```python
from build123d import *

# Parameters (mm, degrees)
F0_W      = 42
F0_H      = 31
F0_R      = 2.25
F0_W_2    = 32
F0_H_2    = 15
F1_DEPTH  = 7
F0_H_3    = 21
F2_DEPTH  = 3
F0_H_4    = 19
F3_DEPTH  = 17
F4_R      = 5
F5_R      = 5
F6_R      = 6.25
F7_DEPTH  = 25
F9_DEPTH  = 3
F11_DEPTH = 3
F12_R     = 1.6772479293
F12_R_2   = 1.75
F13_DEPTH = 25
F6_R_2    = 8.25
F14_DEPTH = 14
F15_R     = 1.625
F16_DEPTH = 30
F17_R     = 2.25
F18_DEPTH = 4


with BuildPart() as f1:
    # F0 (on Top) → F1 (new body)
    with BuildSketch(Plane.XY):
        with Locations((0, -15.5)):
            Rectangle(F0_W, F0_H)
        with Locations((-9.75, -23)):
            Circle(F0_R, mode=Mode.SUBTRACT)
        with Locations((0, -25)):
            Circle(F0_R, mode=Mode.SUBTRACT)
        with Locations((9.75, -23)):
            Circle(F0_R, mode=Mode.SUBTRACT)
        with Locations((0, -10.5)):
            Rectangle(F0_W_2, F0_H_2, mode=Mode.SUBTRACT)
    extrude(amount=F1_DEPTH)



with BuildPart() as f2:
    # F0 (on Top) → F2 (new body)
    with BuildSketch(Plane.XY):
        with Locations((0, 29.5)):
            Rectangle(F0_W, F0_H_3)
        with Locations((-3.5, 33.5)):
            Circle(F0_R, mode=Mode.SUBTRACT)
        with Locations((15, 30.5)):
            Circle(F0_R, mode=Mode.SUBTRACT)
    extrude(amount=F2_DEPTH)


with BuildPart() as f1_1:
    add(f1.part)

    add(f2.part)  # F3 merges F2
    # F0 (on Top) → F3 (join)
    with BuildSketch(Plane.XY):
        with Locations((0, 9.5)):
            Rectangle(F0_W, F0_H_4)
    extrude(amount=F3_DEPTH)

    # F4
    f4_edges = [f1_1.edges().sort_by_distance(p)[0] for p in [
        (-21, -31, 3.5),
        (21, -31, 3.5),
    ]]
    fillet(f4_edges, radius=F4_R)

    # F5
    f5_edges = [f1_1.edges().sort_by_distance(p)[0] for p in [
        (-21, 40, 1.5),
        (21, 40, 1.5),
        (21, 9.5, 17),
        (-21, 9.5, 17),
    ]]
    fillet(f5_edges, radius=F5_R)

    # F6 (on face) → F7 (cut)
    with BuildSketch(Plane(origin=(0, 0, 0), x_dir=(1, 0, 0), z_dir=(0, 0, -1))):
        with Locations((-3.5, -9.5)):
            Circle(F6_R)
    extrude(amount=-F7_DEPTH, mode=Mode.SUBTRACT)

    # F8 (on face) → F9 (join)
    with BuildSketch(Plane(origin=(-21, 0, 0), x_dir=(0, -1, 0), z_dir=(-1, 0, 0))):
        Polygon((-19, 3), (-19, 12), (-26, 3), align=None)
    extrude(amount=-F9_DEPTH)

    # F10 (on face) → F11 (join)
    with BuildSketch(Plane.YZ.offset(21)):
        Polygon((26, 3), (19, 12), (19, 3), align=None)
    extrude(amount=-F11_DEPTH)

    # F12 (on face) → F13 (cut)
    with BuildSketch(Plane.XZ):
        with Locations((-15.5, 13)):
            Circle(F12_R)
        with Locations((15.5, 13)):
            Circle(F12_R_2)
    extrude(amount=-F13_DEPTH, mode=Mode.SUBTRACT)

    # F6 (on face) → F14 (cut)
    with BuildSketch(Plane(origin=(0, 0, 0), x_dir=(1, 0, 0), z_dir=(0, 0, -1))):
        with Locations((-3.5, -9.5)):
            Circle(F6_R_2)
        with Locations((-3.5, -9.5)):
            Circle(F6_R, mode=Mode.SUBTRACT)
    extrude(amount=-F14_DEPTH, mode=Mode.SUBTRACT)

    # F15 (on face) → F16 (cut)
    with BuildSketch(Plane(origin=(0, 19, 0), x_dir=(-1, 0, 0), z_dir=(0, 1, 0))):
        with Locations((-4, 5.1853246987)):
            Circle(F15_R)
        with Locations((11, 5.1853246987)):
            Circle(F15_R)
    extrude(amount=-F16_DEPTH, mode=Mode.SUBTRACT)

    # F17 (on face) → F18 (cut)
    with BuildSketch(Plane.XY.offset(7)):
        Polygon((-5.5006545536, -22.9254126202), (-7.6899218425, -19.2826652041), (-11.9392672889, -19.3572525839), (-13.9993454464, -23.0745873798), (-11.8100781575, -26.7173347959), (-7.5607327111, -26.6427474161), align=None)
        with Locations((-9.75, -23)):
            Circle(F17_R, mode=Mode.SUBTRACT)
        Polygon((4.2483044025, -24.9471547253), (2.0783868508, -21.2944378271), (-2.1699175516, -21.3472831018), (-4.2483044025, -25.0528452747), (-2.0783868508, -28.7055621729), (2.1699175516, -28.6527168982), align=None)
        with Locations((0, -25)):
            Circle(F17_R, mode=Mode.SUBTRACT)
        Polygon((13.9979346939, -22.9229691252), (11.8072566524, -19.2826652041), (7.5593219586, -19.3596960789), (5.5020653061, -23.0770308748), (7.6927433476, -26.7173347959), (11.9406780414, -26.6403039211), align=None)
        with Locations((9.75, -23)):
            Circle(F17_R, mode=Mode.SUBTRACT)
    extrude(amount=-F18_DEPTH, mode=Mode.SUBTRACT)


solid = f1_1.part
```
Check sheet for the modelled part. Datum: model origin and axes. Units: mm. A direction names the side the tool comes from. Give positions to 0.01 mm unless a question says otherwise; leave off trailing zeros. Write each loop counter-clockwise with the first axis right and the second up, starting at its lowest first coordinate (ties: lowest second). Pieces come first, ordered by that corner, then holes. Notation, with made-up numbers: (70, 7) - (78, 7) arc R19 cw to (78, 27) - close; hole circle Ø11 at (47.5, 9). An arc over 180 degrees is marked (long way). Answer as a JSON object with one key per item and string values. Group by question number.
1) Release check for a two-part mould opening along Y. For faces 1 (the face through (-20, 10, 15)), 2 (the face through (-6.6, -21.1, 5)), 3 (the face through (-19.521, 22.451, 7.563)) record: pulls with the +Y half, pulls with the -Y half, needs draft (parallel to the pull), parting line crosses it, or undercut.
2) Depth check by flat-ended pin: P1, Ø2, axis at y = 29, z = 4.5, coming from the -X side; P2, Ø25, axis at x = -0.5, y = -20.5, coming from the +Z side; P3, Ø5, axis at x = -7, y = 29, coming from the +Z side; P4, Ø13, axis at x = -2, y = 9.5, coming from the -Z side. Enter the tip coordinate at first touch or a pass-through.
3) Sectioned sample at C-C (x = -11). Give the number of separate pieces and of enclosed holes in the cut face, then the cut area to 3 significant figures.
4) Sectioned sample at A-A (z = 13). Record the cut outline in (x, y).
5) Thickness scan on probe 1 along Y at (x, z) = (-3.5, 1.25); probe 2 along Y at (x, z) = (15, 1.7); probe 3 along X at (y, z) = (-20, 3.25). Record the ranges inside material, lowest first. Write a range as from..to.
6) Access from +Z, -Z, +X, -X, +Y, -Y to the whole of each face (thin tool, end or side, straight path). Record for faces 4 (the face through (0, -3, 3)), 5 (the face through (3.19, -26.83, 5.03)), 6 (the face through (-5, 3, 14)).
7) Sectioned sample at B-B (y = 30.5). Record the cut outline in (x, z), then the cut area to 4 significant figures.
Geometry results:
{
 "1": {"face 1": "needs draft", "face 2": "undercut", "face 3": "pulls with the +Y half"},
 "2": {"P1": "passes through", "P2": "stops at z = 7", "P3": "stops at z = 3", "P4": "stops at z = 14"},
 "3": {"separate pieces": "5", "enclosed holes": "0", "area": "312 mm^2"},
 "4": {"outline": "(-20.9, 0) - (-17.18, 0) - (-17.18, 19) - (-20.9, 19) - close; (-13.82, 0) - (13.75, 0) - (13.75, 19) - (-13.82, 19) - close; (17.25, 0) - (20.9, 0) - (20.9, 19) - (17.25, 19) - close; hole circle Ø16.5 at (-3.5, 9.5)"},
 "5": {"probe 1": "y = -31..-18, -3..1.25, 17.75..31.25, 35.75..40", "probe 2": "y = -31..-18, -3..28.25, 32.75..40", "probe 3": "x = -21..-12.3, -7.26..7.2, 12.24..21"},
 "6": {"face 4": "+Z, -Z", "face 5": "+Z", "face 6": "-Z"},
 "7": {"outline": "(-21, 0) - (12.75, 0) - (12.75, 3) - (-21, 3) - close; (17.25, 0) - (21, 0) - (21, 3) - (17.25, 3) - close", "area": "112.5 mm^2"}
}
